```python
from build123d import *

# Parameters (mm, degrees)
PAD_DEPTH       = 6
PAD001_DEPTH    = 1
PAD002_DEPTH    = 6
SKETCH003_R     = 13.15
POCKET_DEPTH    = 6
SKETCH004_R     = 13.15
POCKET001_DEPTH = 6
SKETCH005_R     = 12
POCKET002_DEPTH = 1
SKETCH006_W     = 6
SKETCH006_H     = 10
POCKET003_DEPTH = 13


with BuildPart() as part:
    # Sketch → Pad (new body)
    with BuildSketch(Plane.XY):
        with BuildLine():
            Line((-7.317568, 14.228605), (-18, 35))
            Line((-18, 35), (-18, -35))
            Line((-18, -35), (-7.317568, -14.228605))
            ThreePointArc((-7.317568, -14.228605), (16, 0), (-7.317568, 14.228605))
        make_face()
    extrude(amount=PAD_DEPTH)

    # Sketch001 (on Face6 of Pad) → Pad001 (join)
    with BuildSketch(Plane.XY.offset(6)):
        with BuildLine():
            Line((-7.088894, 13.783961), (-18, 35))
            Line((-18, 35), (-18, -35))
            Line((-18, -35), (-7.088894, -13.783961))
            ThreePointArc((-7.088894, -13.783961), (15.5, 0), (-7.088894, 13.783961))
        make_face()
    extrude(amount=PAD001_DEPTH)

    # Sketch002 (on Face10 of Pad001) → Pad002 (join)
    with BuildSketch(Plane.XY.offset(7)):
        with BuildLine():
            Line((-7.317568, 14.228605), (-18, 35))
            Line((-18, 35), (-18, -35))
            Line((-18, -35), (-7.317568, -14.228605))
            ThreePointArc((-7.317568, -14.228605), (16, 0), (-7.317568, 14.228605))
        make_face()
    extrude(amount=PAD002_DEPTH)

    # Sketch003 (on Face4 of Pad002) → Pocket (cut)
    with BuildSketch(Plane(origin=(0, 0, 0), x_dir=(1, 0, 0), z_dir=(0, 0, -1))):
        Circle(SKETCH003_R)
    extrude(amount=-POCKET_DEPTH, mode=Mode.SUBTRACT)

    # Sketch004 (on Face17 of Pocket) → Pocket001 (cut)
    with BuildSketch(Plane.XY.offset(13)):
        Circle(SKETCH004_R)
    extrude(amount=-POCKET001_DEPTH, mode=Mode.SUBTRACT)

    # Sketch005 (on Face20 of Pocket001) → Pocket002 (cut)
    with BuildSketch(Plane.XY.offset(7)):
        Circle(SKETCH005_R)
    extrude(amount=-POCKET002_DEPTH, mode=Mode.SUBTRACT)

    # Sketch006 (on Face17 of Pocket002) → Pocket003 (cut)
    with BuildSketch(Plane.XY.offset(13)):
        with Locations((13, 0)):
            Rectangle(SKETCH006_W, SKETCH006_H)
    extrude(amount=-POCKET003_DEPTH, mode=Mode.SUBTRACT)


solid = part.part
```
For this review, take the finished solid that the model builds, in its own axes (mm). A direction names the side the tool comes from. Coordinates: 2 decimals unless noted, no trailing zeros. Loops run counter-clockwise (first coordinate to the right, second up) from the corner with the lowest first, then second, coordinate; pieces in that order, holes last. Notation, with made-up numbers: (79, -31.5) - (101, -31.5) arc R19 cw to (101, -21.5) - close; hole circle Ø8 at (17.5, 24.5). An arc over 180 degrees is marked (long way). Use one line per item in the form item = value. Start each with the question number.
1) Take a section at A-A (x = 0). State the section outline as (y, z) points.
2) Take a section at C-C (z = 2). State the section outline as (x, y) points.
3) Take a section at B-B (y = 0). State the section outline as (x, z) points, plus the area to 3 significant figures.
4) Take a section at D-D (x = -14). State the section outline as (y, z) points, plus the area to 3 significant figures.
5) To check wall thickness, follow probe 1 along Y at (x, z) = (0, 6.5); probe 2 along Y at (x, z) = (0, 1.65); probe 3 along X at (y, z) = (0, 6.45). State the ranges of each line that lie inside material, in increasing order. Write a range as from..to.
6) For pin 1 (1 mm diameter, centred on x = 7.5, z = 8, fed in from +Y); pin 2 (2 mm diameter, centred on x = 13.5, z = 7.5, fed in from -Y); pin 3 (3 mm diameter, centred on x = -13.5, z = 5.5, fed in from +Y); pin 4 (14.5 mm diameter, centred on x = 0, y = 0, fed in from -Z), all flat-tipped, find the tip position at first contact; note any pin that passes through.
7) Draft analysis for pull direction X (two halves, no side actions). For faces 1 (the face through (-18, 0, 6)), 2 (the face through (6.25, 14.73, 2.96)), 3 (the face through (-14, 0, 13)), state which applies: released by +X, released by -X, zero draft, split by the parting line, or undercut.
8) For faces 4 (the face through (-13.14, -0.51, 2.96)), 5 (the face through (-12, -3, 7)), 6 (the face through (5.974, 14.302, 6.493)), 7 (the face through (14, -5, 7)), 8 (the face through (5.63, -14.44, 6.49)), list the 3-axis set-ups (+Z, -Z, +X, -X, +Y, -Y) from which the entire face can be reached by the end or side of a thin tool; tool diameter is ignored.
From the geometry:
q1.outline = (-16, 0) - (-13.15, 0) - (-13.15, 6) - (-12, 6) - (-12, 7) - (-13.15, 7) - (-13.15, 13) - (-16, 13) - (-16, 7) - (-15.5, 7) - (-15.5, 6) - (-16, 6) - close; (12, 6) - (13.15, 6) - (13.15, 0) - (16, 0) - (16, 6) - (15.5, 6) - (15.5, 7) - (16, 7) - (16, 13) - (13.15, 13) - (13.15, 7) - (12, 7) - close
q2.outline = (-18, -35) - (-7.32, -14.23) arc R16 ccw to (15.2, -5) - (12.16, -5) arc R13.15 cw (long way) to (12.16, 5) - (15.2, 5) arc R16 ccw to (-7.32, 14.23) - (-18, 35) - close
q3.outline = (-18, 0) - (-13.15, 0) - (-13.15, 6) - (-12, 6) - (-12, 7) - (-13.15, 7) - (-13.15, 13) - (-18, 13) - close
q3.area = 64.2 mm2
q4.outline = (-27.22, 0) - (27.22, 0) - (27.22, 13) - (-27.22, 13) - close
q4.area = 708 mm2
q5.probe_1 = -15.5..-12, 12..15.5
q5.probe_2 = -16..-13.15, 13.15..16
q5.probe_3 = -18..-12
q6.pin_1 = 14.39
q6.pin_2 = -9.99
q6.pin_3 = 29.17
q6.pin_4 = through
q7.face_1 = released by -X
q7.face_2 = undercut
q7.face_3 = zero draft
q8.face_4 = -Z
q8.face_5 = +Z
q8.face_6 = +Y
q8.face_7 = +Z, -Z, +X
q8.face_8 = -Y
